```python
from build123d import *

# Parameters (mm, degrees)
F0_R     = 24.5
F0_W     = 4
F0_H     = 3
F0_R_2   = 1.5
F0_W_2   = 6
F1_DEPTH = 0.3
F2_DEPTH = 1.5


with BuildPart() as f1:
    # F0 (on Top) → F1 (new body)
    with BuildSketch(Plane.XY):
        Circle(F0_R)
        Polygon((-4.75, -4.75), (-4.75, 4.75), (4.75, 4.75), (4.75, -4.75), (3, -4.75), (3, -7.75), (4, -7.75), (4, -13.75), (-4, -13.75), (-4, -7.75), (-3, -7.75), (-3, -4.75), align=None, mode=Mode.SUBTRACT)
        with Locations((7, -10.25)):
            Rectangle(F0_W, F0_H, mode=Mode.SUBTRACT)
        with Locations((-10.5, 0.5)):
            Circle(F0_R_2, mode=Mode.SUBTRACT)
        with Locations((10.5, 0.5)):
            Circle(F0_R_2, mode=Mode.SUBTRACT)
        with Locations((7, -10.25)):
            Rectangle(F0_W, F0_H)
        Polygon((3, -7.75), (-3, -7.75), (-4, -7.75), (-4, -13.75), (4, -13.75), (4, -7.75), align=None)
        with Locations((0, -6.25)):
            Rectangle(F0_W_2, F0_H)
    extrude(amount=F1_DEPTH)

    # F0 (on Top) → F2 (join)
    with BuildSketch(Plane.XY):
        Circle(F0_R)
        Polygon((-4.75, -4.75), (-4.75, 4.75), (4.75, 4.75), (4.75, -4.75), (3, -4.75), (3, -7.75), (4, -7.75), (4, -13.75), (-4, -13.75), (-4, -7.75), (-3, -7.75), (-3, -4.75), align=None, mode=Mode.SUBTRACT)
        with Locations((7, -10.25)):
            Rectangle(F0_W, F0_H, mode=Mode.SUBTRACT)
        with Locations((-10.5, 0.5)):
            Circle(F0_R_2, mode=Mode.SUBTRACT)
        with Locations((10.5, 0.5)):
            Circle(F0_R_2, mode=Mode.SUBTRACT)
    extrude(amount=F2_DEPTH)


solid = f1.part
```
Geometry check sheet. Reference: the model listing, model coordinates, mm. A direction names the side the tool comes from. Give positions to 0.01 mm unless a question says otherwise; leave off trailing zeros. Write each loop counter-clockwise with the first axis right and the second up, starting at its lowest first coordinate (ties: lowest second). Pieces come first, ordered by that corner, then holes. Notation, with made-up numbers: (17.25, 13) -> (64.25, 13) arc R19 cw to (64.25, 47) -> close; hole circle Ø7 at (42.25, 86.5). An arc over 180 degrees is marked (long way). Use one line per item in the form item = value.
Item 1: Sectioned sample at A-A on z = 1.05. Enter the section's corners in (x, y).
Results list:
outline = circle Ø49 at (0, 0); hole circle Ø3 at (-10.5, 0.5); hole (-4.75, -4.75) -> (-3, -4.75) -> (-3, -7.75) -> (-4, -7.75) -> (-4, -13.75) -> (4, -13.75) -> (4, -7.75) -> (3, -7.75) -> (3, -4.75) -> (4.75, -4.75) -> (4.75, 4.75) -> (-4.75, 4.75) -> close; hole (5, -11.75) -> (9, -11.75) -> (9, -8.75) -> (5, -8.75) -> close; hole circle Ø3 at (10.5, 0.5)
Item 2: Sectioned sample at C-C on y = -6. Enter the section's corners in (x, z), plus the area to 3 significant figures.
Results list:
outline = (-23.75, 0) -> (23.75, 0) -> (23.75, 1.5) -> (3, 1.5) -> (3, 0.3) -> (-3, 0.3) -> (-3, 1.5) -> (-23.75, 1.5) -> close
area = 64.1 mm2
Item 3: Depth check by flat-ended pin: pin 1 Ø0.6 at (y, z) = (-10, 1) entering from -X; pin 2 Ø0.8 at (x, z) = (-1.5, 0.5) entering from -Y. Enter the tip coordinate at first touch or a pass-through.
Results list:
pin_1 = -22.5
pin_2 = -24.48
Item 4: Sectioned sample at D-D on x = -10.5. Enter the section's corners in (y, z), plus the area to 3 significant figures.
Results list:
outline = (-22.14, 0) -> (-1, 0) -> (-1, 1.5) -> (-22.14, 1.5) -> close; (2, 0) -> (22.14, 0) -> (22.14, 1.5) -> (2, 1.5) -> close
area = 61.9 mm2
Item 5: Scan lines: line 1 (X direction, y = -11.5, z = 0.95); line 2 (Y direction, x = 10.5, z = 0.55); line 3 (Y direction, x = -2.5, z = 0.5). Record each from-to range of solid material in increasing order.
Results list:
line_1 = -21.63 to -4, 4 to 5, 9 to 21.63
line_2 = -22.14 to -1, 2 to 22.14
line_3 = -24.37 to -13.75, 4.75 to 24.37
Item 6: Access from +Z, -Z, +X, -X, +Y, -Y to the whole of each face (thin tool, end or side, straight path). Record for faces 4 (the flat face through (0, 4.75, 1)), 5 (the flat face through (0, -5, 0)), 6 (the flat face through (9, -10, 1)).
Results list:
face_4 = +Z, -Z
face_5 = -Z, +X, -X, +Y, -Y
face_6 = +Z
Item 7: Sectioned sample at B-B on x = -0.5. Enter the section's corners in (y, z), plus the area to 3 significant figures.
Results list:
outline = (-24.49, 0) -> (-4.75, 0) -> (-4.75, 0.3) -> (-13.75, 0.3) -> (-13.75, 1.5) -> (-24.49, 1.5) -> close; (4.75, 0) -> (24.49, 0) -> (24.49, 1.5) -> (4.75, 1.5) -> close
area = 48.4 mm2
Item 8: Mould release check, pull along X, two halves, no side actions. Record for faces 1 (the cylindrical face through (13.17, 20.66, 0.74)), 2 (the flat face through (7, -8.75, 1)), 3 (the flat face through (5, 0, 1.5)): released by +X, released by -X, zero draft, split by the parting line, or undercut.
Results list:
face_1 = split by the parting line
face_2 = undercut
face_3 = zero draft
